Could you check a few things on this drawing? It's one solid part, dimensions in mm from its lowest x, y, z. Coordinates: 2 decimals unless noted, no trailing zeros. Order: outer loops, then holes, each group sorted by start corner. A loop starts at its lowest first (then second) coordinate and runs counter-clockwise, first axis right, second up. Notation, with made-up numbers: (-20.5, 7.25) - (19.5, 7.25) arc R15 cw to (19.5, 12.25) - close; hole circle Ø7 at (-39.5, 9). An arc over 180 degrees is marked (long way). Answer in a Markdown table with one row per item. Add a question column.
Item 1: I want a section at D-D (y = 2.25). Count the separate pieces of the cut face and the enclosed holes in it, plus the area to 3 significant figures.
Item 2: If I drill on line 1 along Z through (x, y) = (157.5, 11.25) (1 decimal); line 2 along X through (y, z) = (3.5, 177.5) (1 decimal); line 3 along Z through (x, y) = (233, 9) (1 decimal), over which ranges is the centre line in solid material (lowest first)? Write a range as from..to.
Item 3: Will these pins go through, and if not, where does the flat tip stop? pin 1 Ø1.5 at (y, z) = (10.5, 195) entering from +X; pin 2 Ø5 at (x, y) = (59, 4.5) entering from +Z; pin 3 Ø2 at (y, z) = (5.5, 122) entering from +X.
Item 4: I want a section at C-C (z = 279.4). Please give me the cut outline in (x, y).
Item 5: I want a section at A-A (z = 152.4). Please give me the cut outline in (x, y), plus the area to 3 significant figures.
Item 6: Thinking about a two-plate mould opening in Y: for the marked faces 1 and 2, which applies, +Y half, -Y half, draft (parallel to the pull), parting line (faces both ways), or undercut?
Item 7: I want a section at B-B (x = 279.4). Please give me the cut outline in (y, z), plus the area to 3 significant figures.
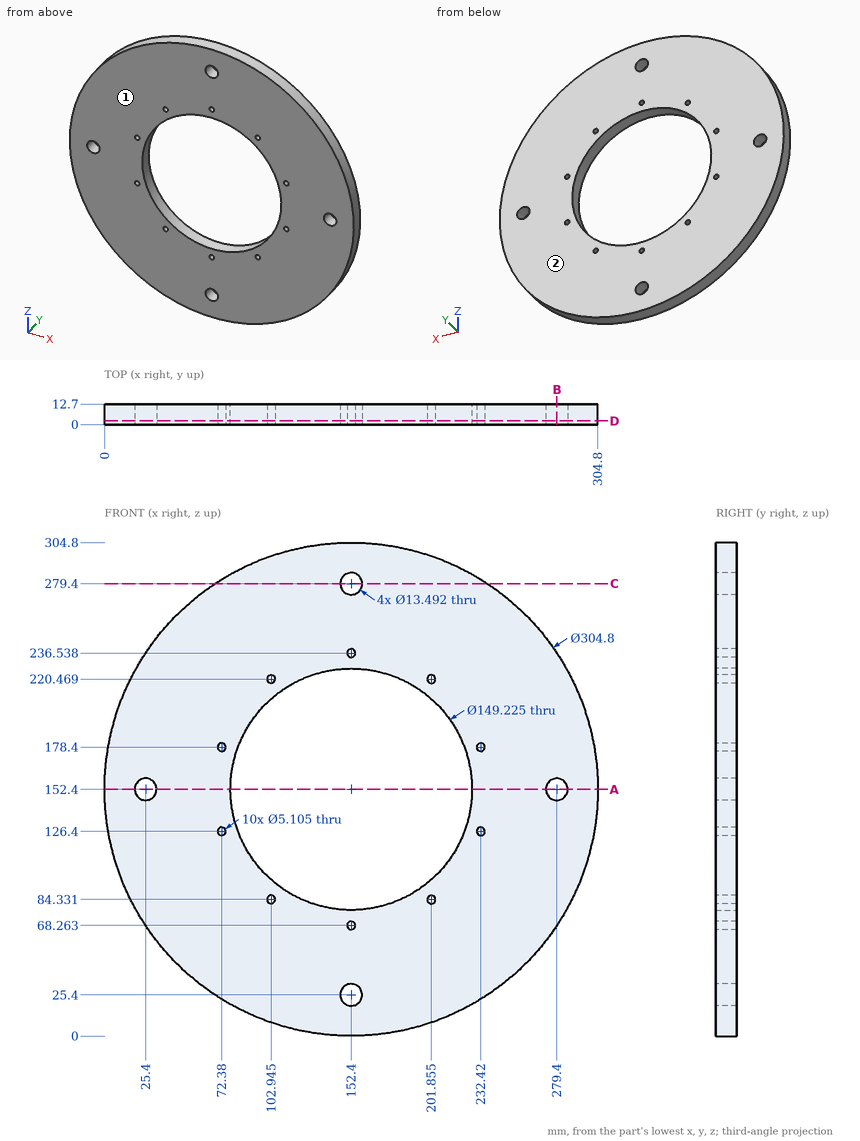
Values follow:
| question | item | result |
|---|---|---|
| 1 | separate pieces | 1 |
| 1 | enclosed holes | 15 |
| 1 | area | 54,700 mm^2 |
| 2 | line 1 | z = 0.1..21, 29.8..78, 226.8..275, 283.8..304.7 |
| 2 | line 2 | x = 2.1..70, 74.8..82.1, 222.7..230, 234.8..302.7 |
| 2 | line 3 | z = 23.1..123.9, 128.9..175.9, 180.9..281.7 |
| 3 | pin 1 | stops at x = 298.94 |
| 3 | pin 2 | stops at z = 274.72 |
| 3 | pin 3 | stops at x = 301.94 |
| 4 | outline | (68.16, 0) - (145.65, 0) - (145.65, 12.7) - (68.16, 12.7) - close; (159.15, 0) - (236.64, 0) - (236.64, 12.7) - (159.15, 12.7) - close |
| 5 | outline | (0, 0) - (18.65, 0) - (18.65, 12.7) - (0, 12.7) - close; (32.15, 0) - (77.79, 0) - (77.79, 12.7) - (32.15, 12.7) - close; (227.01, 0) - (272.65, 0) - (272.65, 12.7) - (227.01, 12.7) - close; (286.15, 0) - (304.8, 0) - (304.8, 12.7) - (286.15, 12.7) - close |
| 5 | area | 1,630 mm^2 |
| 6 | face 1 | -Y half |
| 6 | face 2 | +Y half |
| 7 | outline | (0, 68.16) - (12.7, 68.16) - (12.7, 145.65) - (0, 145.65) - close; (0, 159.15) - (12.7, 159.15) - (12.7, 236.64) - (0, 236.64) - close |
| 7 | area | 1,970 mm^2 |
